Autodesk Fusion 360 part; units mm, degrees
sketch "dino" plane through (0, 0, 0) normal (0, 0, 1) x (1, 0, 0)
  line L0 (-1, -5) -> (-41, -5)
  line L1 (-41, -5) -> (-41, 35)
  line L2 (-41, 35) -> (-1, 35)
  line L3 (-1, 35) -> (-1, -5)
  line L4 (-37.8669, -1.9758) -> (-36, -1.9758)
  line L5 (-36, -1.9758) -> (-36, -3.7206)
  line L6 (-36, -3.7206) -> (-25.1685, -3.7206)
  line L7 (-25.1685, -3.7206) -> (-25.1685, -1.9758)
  line L8 (-25.1685, -1.9758) -> (-23.3, -1.9758)
  line L9 (-23.3, -1.9758) -> (-23.3, 10.7954)
  line L10 (-23.3, 10.7954) -> (-21.5, 10.7954)
  line L11 (-21.5, 10.7954) -> (-21.5, 12.5)
  line L12 (-21.5, 12.5) -> (-19.672, 12.5)
  line L13 (-19.672, 12.5) -> (-19.672, 14.5)
  line L14 (-19.672, 14.5) -> (-17.9, 14.5)
  line L15 (-17.9, 14.5) -> (-17.9, 16.1)
  line L16 (-17.9, 16.1) -> (-16, 16.1)
  line L17 (-16, 16.1) -> (-16, 18)
  line L18 (-16, 18) -> (-14.189, 18)
  line L19 (-14.189, 18) -> (-14.189, 19.764)
  line L20 (-14.189, 19.764) -> (-12.5, 19.764)
  line L21 (-12.5, 19.764) -> (-12.5, 21.5)
  line L22 (-12.5, 21.5) -> (-8.8798, 21.5)
  line L23 (-8.8798, 21.5) -> (-8.8798, 19.764)
  line L24 (-8.8798, 19.764) -> (-7, 19.764)
  line L25 (-7, 19.764) -> (-7, 17.9)
  line L26 (-7, 17.9) -> (-5.1831, 17.9)
  line L27 (-5.1831, 17.9) -> (-5.1831, 16.1484)
  line L28 (-5.1831, 16.1484) -> (-3.2862, 16.1484)
  line L29 (-3.2862, 16.1484) -> (-3.2862, 21.5)
  line L30 (-3.2862, 21.5) -> (-5.1831, 21.5)
  line L31 (-5.1831, 21.5) -> (-5.1831, 25.233)
  line L32 (-5.1831, 25.233) -> (-7, 25.233)
  line L33 (-7, 25.233) -> (-7, 27)
  line L34 (-7, 27) -> (-10.5, 27)
  line L35 (-10.5, 27) -> (-10.5, 29)
  line L36 (-10.5, 29) -> (-12.276, 29)
  line L37 (-12.276, 29) -> (-12.276, 34.5)
  line L38 (-12.276, 34.5) -> (-16, 34.5)
  line L39 (-16, 34.5) -> (-16, 32.5)
  line L40 (-16, 32.5) -> (-14.3257, 32.5)
  line L41 (-14.3257, 32.5) -> (-14.3257, 30.7993)
  line L42 (-14.3257, 30.7993) -> (-16, 30.7993)
  line L43 (-16, 30.7993) -> (-16, 29)
  line L44 (-16, 29) -> (-17.8539, 29)
  line L45 (-17.8539, 29) -> (-17.8539, 30.7993)
  line L46 (-17.8539, 30.7993) -> (-19.6941, 30.7993)
  line L47 (-19.6941, 30.7993) -> (-19.6941, 34.5)
  line L48 (-19.6941, 34.5) -> (-23.2983, 34.5)
  line L49 (-23.2983, 34.5) -> (-23.2983, 32.5)
  line L50 (-23.2983, 32.5) -> (-21.4962, 32.5)
  line L51 (-21.4962, 32.5) -> (-21.4962, 25.308)
  line L52 (-21.4962, 25.308) -> (-23.2983, 25.308)
  line L53 (-23.2983, 25.308) -> (-23.2983, 21.6664)
  line L54 (-23.2983, 21.6664) -> (-25.1992, 21.6664)
  line L55 (-25.1992, 21.6664) -> (-25.1992, 18)
  line L56 (-25.1992, 18) -> (-27, 18)
  line L57 (-27, 18) -> (-27, 16.1853)
  line L58 (-27, 16.1853) -> (-30.633, 16.1853)
  line L59 (-30.633, 16.1853) -> (-30.633, 7)
  line L60 (-30.633, 7) -> (-36, 7)
  line L61 (-36, 7) -> (-36, 5.2364)
  line L62 (-36, 5.2364) -> (-30.633, 5.2364)
  line L63 (-30.633, 5.2364) -> (-30.633, 3.5)
  line L64 (-30.633, 3.5) -> (-37.8295, 3.5)
  line L65 (-37.8295, 3.5) -> (-37.8669, -1.9758)
  line L66 (-30.6, -1.9) -> (-28.9, -1.9)
  line L67 (-28.9, -1.9) -> (-28.9, -0.2)
  line L68 (-28.9, -0.2) -> (-30.633, -0.2)
  line L69 (-30.633, -0.2) -> (-30.6, -1.9)
  line L70 (-30.633, 12.6033) -> (-28.9, 12.6033)
  line L71 (-28.9, 12.6033) -> (-28.9, 14.2784)
  line L72 (-28.9, 14.2784) -> (-34.5, 14.2784)
  line L73 (-34.5, 14.2784) -> (-34.5, 18)
  line L74 (-34.5, 18) -> (-32.5, 18)
  line L75 (-32.5, 18) -> (-32.5, 16.1392)
  line L76 (-32.5, 16.1392) -> (-30.633, 16.1853)
  line L77 (-30.633, 17.9928) -> (-28.8165, 17.9928)
  line L78 (-28.8165, 17.9928) -> (-28.8165, 21.5)
  line L79 (-28.8165, 21.5) -> (-27, 21.5)
  line L80 (-27, 21.5) -> (-27, 23.5)
  line L81 (-27, 23.5) -> (-25.274, 23.5)
  line L82 (-25.274, 23.5) -> (-25.274, 25.1824)
  line L83 (-25.274, 25.1824) -> (-23.5, 25.1824)
  line L84 (-23.5, 25.1824) -> (-23.5, 27)
  line L85 (-23.5, 27) -> (-21.4962, 27)
  line L86 (-30.633, 17.9928) -> (-30.633, 16.1853)
  dimension "d1" = 40
  dimension "d2" = 40
extrude "Extrude1" add sketch "dino" along normal blind 3 contours L4 L5 L6 L7 L8 L9 L10 L11 L12 L13 L14 L15 L16 L17 L18 L19 L20 L21 L22 L23 L24 L25 L26 L27 L28 L29 L30 L31 L32 L33 L34 L35 L36 L37 L38 L39 L40 L41 L42 L43 L44 L45 L46 L47 L48 L49 L50 L51 L52 L53 L54 L55 L56 L57 L58 L59 L60 L61 L62 L63 L64 L65 L70 L71 L72 | L59 L72 L73 L74 L75 L76
extrude "Extrude2" add sketch "dino" along normal blind 2 and the other way blind -1 contours L59 L70 L71 L72 | L51 L52 L53 L54 L55 L56 L57 L58 L77 L78 L79 L80 L81 L82 L83 L84 L85 L86
Model file for the job. Use its own axes, mm. A direction names the side the tool comes from. Give positions to 0.01 mm unless a question says otherwise; leave off trailing zeros. Order: outer loops, then holes, each group sorted by start corner. A loop starts at its lowest first (then second) coordinate and runs counter-clockwise, first axis right, second up. Notation, with made-up numbers: (21, 77) -> (32, 77) arc R28 cw to (32, 116) -> close; hole circle Ø2 at (73.25, -24). An arc over 180 degrees is marked (long way). Use CSV: the item, a comma, the result in double quotes.
1. Mould opens along X. For faces 4 (the flat face through (-30, 13, 2)), 5 (the flat face through (-14.189, 19, 1)), 6 (the flat face through (-25.199, 19.9, 0.5)) say: +X half, -X half, draft (parallel to the pull), parting line (faces both ways), or undercut.
Outcome:
face 4,"draft"
face 5,"undercut"
face 6,"-X half"
2. 3-axis set-ups, long thin cutter, end or side, ignore diameter. For faces 1 (the flat face through (-27, 17.1, 2.5)), 2 (the flat face through (-29.8, 12.603, 0.5)), 3 (the flat face through (-34, 18, 1)): which of +Z, -Z, +X, -X, +Y, -Y reach the whole face in a straight line?
Outcome:
face 1,"+Z, +Y"
face 2,"-Z, -X"
face 3,"+Z, -Z, -X, +Y"
3. Drop flat-ended pins along their axis: pin 1 (2 mm diameter, centred on x = -21.5, y = 27, fed in from -Z); pin 2 (0.5 mm diameter, centred on y = 20.5, z = 1.5, fed in from -X); pin 3 (0.5 mm diameter, centred on x = -30, z = 1.5, fed in from +Y); pin 4 (0.8 mm diameter, centred on x = -30, z = 2.5, fed in from +Y). Give the stop position or say it passes through.
Outcome:
pin 1,"z = 0"
pin 2,"x = -28.82"
pin 3,"y = 17.99"
pin 4,"y = 16.19"
4. Band-saw the part on D-D, the plane x = -11.5. Give the cut face in (y, z).
Outcome:
outline,"(21.5, 0) -> (29, 0) -> (29, 3) -> (21.5, 3) -> close"
5. Band-saw the part on C-C, the plane y = 6. Give the cut face in (x, z).
Outcome:
outline,"(-36, 0) -> (-23.3, 0) -> (-23.3, 3) -> (-36, 3) -> close"
6. Band-saw the part on A-A, the plane y = 17. Give the cut face in (x, z), then the cut area to 3 significant figures.
Outcome:
outline,"(-34.5, 0) -> (-32.5, 0) -> (-32.5, 3) -> (-34.5, 3) -> close; (-30.63, 1) -> (-27, 1) -> (-27, 0) -> (-16, 0) -> (-16, 3) -> (-27, 3) -> (-27, 2) -> (-30.63, 2) -> close; (-5.18, 0) -> (-3.29, 0) -> (-3.29, 3) -> (-5.18, 3) -> close"
area,"48.3 mm²"
7. Band-saw the part on B-B, the plane x = -22.5. Give the cut face in (y, z).
Outcome:
outline,"(10.8, 0) -> (25.31, 0) -> (25.31, 1) -> (27, 1) -> (27, 2) -> (25.31, 2) -> (25.31, 3) -> (10.8, 3) -> close; (32.5, 0) -> (34.5, 0) -> (34.5, 3) -> (32.5, 3) -> close"
8. Drill centre lines: line 1 along X through (y, z) = (17, 2.1); line 2 along Y through (x, z) = (-33, 2); line 3 along Y through (x, z) = (-32, 2.3). Where is each one in solid material? Low to high. Write a range as from..to.
Outcome:
line 1,"-34.5..-32.5, -27..-16, -5.18..-3.29"
line 2,"-3.72..3.5, 5.24..7, 14.28..18"
line 3,"-3.72..3.5, 5.24..7, 14.28..16.15"
